Read the model definition and answer for the solid it produces. Units are mm, in the model's axes. Coordinates: 2 decimals unless noted, no trailing zeros. Loops run counter-clockwise (first coordinate to the right, second up) from the corner with the lowest first, then second, coordinate; pieces in that order, holes last. Notation, with made-up numbers: (-25.5, -7.5) - (-2.5, -7.5) arc R18 ccw to (-2.5, 5.5) - close; hole circle Ø1 at (-27, 28.5). An arc over 180 degrees is marked (long way). One line per item, written item: value. Start each with the question number.
from build123d import *

# Parameters (mm, degrees)
PAD002_DEPTH           = 70
SKETCH006_R            = 6
POCKET002_DEPTH        = 30
SKETCH007_R            = 6
POCKET003_DEPTH        = 343.6422176588
LINEARPATTERN001_COUNT = 4
LINEARPATTERN001_PITCH = 200


with BuildPart() as part:
    # Sketch004 → Pad002 (new body)
    with BuildSketch(Plane.XY):
        with BuildLine():
            Line((-547.6857118143, 425), (19.5015988359, 27.8511695058))
            ThreePointArc((34, 0), (30.1583683281, 15.69945285), (19.5015988359, 27.8511695058))
            Line((24, 0), (34, 0))
            ThreePointArc((24, 0), (21.2882599963, 11.0819667176), (13.7658344724, 19.6596490629))
            Line((13.7658344724, 19.6596490629), (-553.4214761778, 416.8084795571))
            Line((-553.4214761778, 416.8084795571), (-547.6857118143, 425))
        make_face()
    extrude(amount=PAD002_DEPTH)

    # Sketch006 → Pocket002 (cut)
    with BuildSketch(Plane(origin=(0, 126.75, 0), x_dir=(-1, 0, 0), z_dir=(0, 1, 0))):
        with Locations((26.7405688034, 25.24131)):
            Circle(SKETCH006_R)
    extrude(amount=-POCKET002_DEPTH, mode=Mode.SUBTRACT)

    # Sketch007 (on Face2 of Pocket002) → Pocket003 (cut, through all)
    with BuildSketch(Plane(origin=(13.7658344724, 19.6596490629, 0), x_dir=(0.8191520443, -0.5735764364, 0), z_dir=(-0.5735764364, -0.8191520443, 0))):
        with Locations((-672.4078559097, 45)):
            Circle(SKETCH007_R)
    pocket003 = extrude(amount=-POCKET003_DEPTH, mode=Mode.SUBTRACT)

    # LinearPattern001: Pocket003 ×4
    with Locations(*[Vector(0.8191520443, -0.5735764364, 0) * (i * LINEARPATTERN001_PITCH) for i in range(1, LINEARPATTERN001_COUNT)]):
        add(pocket003, mode=Mode.SUBTRACT)

    # Mirrored001: part across XZ


with BuildPart() as part_1:
    add(part.part)
    add(part.part.mirror(Plane.XZ))


with BuildPart() as part_2:
    # Body001 placement: moved
    add(part_1.part.moved(Location((0, 0, -20))))


solid = part_2.part
1) Section A-A, the plane x = -244 is taken. Determine the outline of the cut face in (y, z), and give its area (3 significant figures).
2) Section C-C, the plane y = 198.5 is taken. Determine the outline of the cut face in (x, z), and give its area (3 significant figures).
3) Straight lines are drawn through the part: L1, parallel to Y at x = -113, z = -9; L2, parallel to Y at x = 8, z = 8.5; L3, parallel to X at y = -2, z = 19. For each, find the intervals that lie inside material, in ascending order.
4) Determine the mould class of faces 1 (the flat face through (-268.062, -229.206, 14.51)), 2 (the flat face through (-265.858, 215.454, 14.51)), 3 (the flat face through (-265.858, -215.454, 14.51)), 4 (the flat face through (-268.062, 229.206, 14.51)) for opening direction Y: released by +Y, released by -Y, zero draft, split by the parting line, or undercut.
5) Flat-ended cylindrical pins translate along their axes: P1, Ø1, axis at x = -260, z = 19.5, coming from the +Y side; P2, Ø10, axis at y = -23, z = 4.5, coming from the -X side; P3, Ø10, axis at x = -85, z = 19, coming from the -Y side (3 decimals). Find the tip coordinate at first contact, or state that the pin passes through.
6) Section B-B, the plane z = 2 is taken. Determine the outline of the cut face in (x, y).
Answer below:
1. outline: (-212.36, -20) - (-200.15, -20) - (-200.15, 50) - (-212.36, 50) - close; (200.15, -20) - (212.36, -20) - (212.36, 50) - (200.15, 50) - close
1. area: 1,710 mm2
2. outline: (-241.64, -20) - (-224.21, -20) - (-224.21, 50) - (-241.64, 50) - close
2. area: 1,220 mm2
3. L1: -120.63 to -108.42, 108.42 to 120.63
3. L2: -35.9 to -23.7, 23.7 to 35.9
3. L3: 23.92 to 33.94
4. face 1: released by -Y
4. face 2: undercut
4. face 3: undercut
4. face 4: released by +Y
5. P1: y = 223.91
5. P2: x = 1.85
5. P3: y = -104.525
6. outline: (-553.42, -416.81) - (-547.69, -425) - (19.5, -27.85) arc R34 ccw to (19.5, 27.85) - (-547.69, 425) - (-553.42, 416.81) - (13.77, 19.66) arc R24 cw to (13.77, -19.66) - close
